from build123d import *

# Parameters (mm, degrees)
F3_R     = 5
F5_DEPTH = 5


with BuildPart() as f2:
    # F2: sweep along a path in F1
    with BuildLine(Plane.YZ) as f2_path:
        Line((13.7373713946, 0), (13.7373713946, 15))
        Line((13.7373713946, 15), (-46.2626286054, 15))
    # F0 (on Top) → F2 (sweep)
    with BuildSketch(Plane.XY):
        Polygon((-2.3094010768, 16.5802386344), (-4.6188021535, 12.5802386344), (-2.3094010768, 8.5802386344), (2.3094010768, 8.5802386344), (4.6188021535, 12.5802386344), (2.3094010768, 16.5802386344), align=None)
    sweep(path=f2_path.line, transition=Transition.RIGHT)

    # F3
    f3_edges = [f2.edges().sort_by_distance(p)[0] for p in [
        (0, 16.580239, 17.842867),
    ]]
    fillet(f3_edges, radius=F3_R)

    # F4 (on Right) → F5 (join, symmetric)
    with BuildSketch(Plane.YZ):
        with BuildLine():
            Line((-69.568253388, 8.7428672398), (-82.8082496115, 8.7428672398))
            ThreePointArc((-82.8082496115, 8.7428672398), (-68.9942863231, -0.6953621624), (-56, 9.8428672398))
            Line((-56, 9.8428672398), (-46, 9.8428672398))
            Line((-46, 9.8428672398), (-46, 17.8428672398))
            Line((-46, 17.8428672398), (-56.3282571644, 17.8428672398))
            ThreePointArc((-56.3282571644, 17.8428672398), (-69.568253388, 27.2928672398), (-82.8082496115, 17.8428672398))
            Line((-82.8082496115, 17.8428672398), (-69.568253388, 17.8428672398))
            Line((-69.568253388, 17.8428672398), (-69.568253388, 8.7428672398))
        make_face()
    extrude(amount=F5_DEPTH, both=True)


solid = f2.part
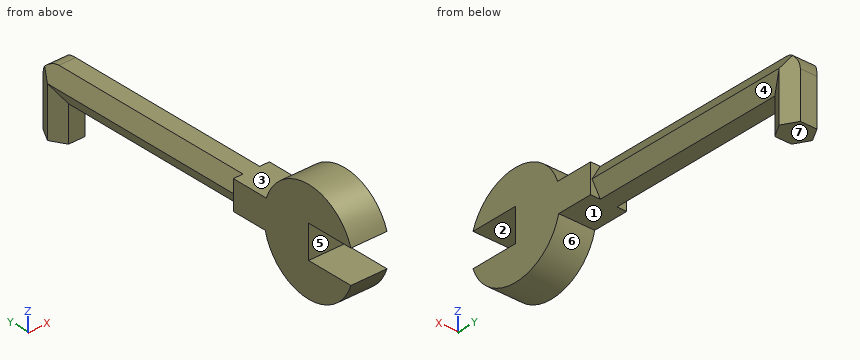
Input: part model. Units: mm. Frame: model coordinates. Face numbers are marked on the shaded views. A direction names the side the tool comes from. Give positions to 0.01 mm unless a question says otherwise; leave off trailing zeros. Write each loop counter-clockwise with the first axis right and the second up, starting at its lowest first coordinate (ties: lowest second). Pieces come first, ordered by that corner, then holes.
Q1. Pull-direction query (Y, two-part tool) for the marked faces 5, 6 and 7; classes: pulls with the +Y half, pulls with the -Y half, needs draft (parallel to the pull), parting line crosses it, or undercut.
Q2. Section D-D, the plane z = 11.5. Output: boundary loops of the cut face in (x, y), plus the area to 3 significant figures.
Q3. Section B-B, the plane x = -0.75. Output: boundary loops of the cut face in (y, z).
Q4. Set-up query: the marked faces 1, 2, 3 and 4. Return all of +Z, -Z, +X, -X, +Y, -Y with unobstructed straight access to the full face (end or side cutting, diameter ignored); none if empty.
Q5. Section A-A, the plane y = -76.5. Output: boundary loops of the cut face in (x, z).
Q6. Material intervals for probe 1 along Y at (x, z) = (2.25, 1); probe 2 along Y at (x, z) = (1, 12.75); probe 3 along Y at (x, z) = (3.25, 7.5), sorted ascending.
Q7. Section C-C, the plane z = 7.5. Output: boundary loops of the cut face in (x, y), plus the area to 3 significant figures.
Q8. First-contact query: P1, Ø3.5, axis at x = -1, z = 6.5, coming from the -Y side; P2, Ø5, axis at x = -0.5, y = -73.5, coming from the -Z side; P3, Ø5, axis at x = 2.5, y = -11, coming from the +Z side. Flat tips, straight axial feed; report the tip coordinate or a pass-through.
Filled in:
1. face 5: pulls with the -Y half
1. face 6: undercut
1. face 7: needs draft
2. outline: (-5, -69.57) - (5, -69.57) - (5, -46) - (3.27, -46) - (3.27, 10.24) - (4.62, 12.58) - (2.31, 16.58) - (-2.31, 16.58) - (-4.62, 12.58) - (-3.27, 10.24) - (-3.27, -46) - (-5, -46) - close
2. area: 649 mm2
3. outline: (-82.81, 8.74) arc R14 ccw to (-56, 9.84) - (8.58, 9.84) - (8.58, 0) - (16.58, 0) - (16.58, 12.84) arc R5 ccw to (11.58, 17.84) - (-56.33, 17.84) arc R14 ccw to (-82.81, 17.84) - (-69.57, 17.84) - (-69.57, 8.74) - close
4. face 1: -Z, +X, -X
4. face 2: +X, -X, -Y
4. face 3: +Z, +X, -X, +Y
4. face 4: -Z, +X
5. outline: (-5, 1.13) - (5, 1.13) - (5, 8.74) - (-5, 8.74) - close; (-5, 17.84) - (5, 17.84) - (5, 25.46) - (-5, 25.46) - close
6. probe 1: y = -76.27 to -62.87, 8.58 to 16.58
6. probe 2: y = -69.57 to 16.58
6. probe 3: y = -82.31 to -56.82, 10.21 to 14.95
7. outline: (-5, -82.31) - (5, -82.31) - (5, -56.82) - (-5, -56.82) - close; (-4.62, 12.58) - (-2.31, 8.58) - (2.31, 8.58) - (4.62, 12.58) - (2.31, 16.58) - (-2.31, 16.58) - close
7. area: 310 mm2
8. P1: stops at y = -82.63
8. P2: stops at z = -0.63
8. P3: stops at z = 17.84
